```python
from build123d import *

# Parameters (mm, degrees)
F0_W     = 50.8
F0_H     = 50.8
F1_DEPTH = 50.8
F3_DEPTH = 25.4
F4_R     = 12.7
F5_DEPTH = 25.4
F6_R     = 12.7
F7_DEPTH = 25.4


with BuildPart() as f1:
    # F0 (on Front) → F1 (new body)
    with BuildSketch(Plane.XZ):
        with Locations((-25.4, 25.4)):
            Rectangle(F0_W, F0_H)
    extrude(amount=F1_DEPTH)

    # F2 (on face) → F3 (join)
    with BuildSketch(Plane.XZ.offset(50.8)):
        Polygon((-12.7, 38.1), (-38.1, 38.1), (-38.1, 10.884415), (-12.984917, 10.884415), align=None)
    extrude(amount=F3_DEPTH)

    # F4 (on face) → F5 (join)
    with BuildSketch(Plane.YZ):
        with Locations((-25.738167, 25.206015)):
            Circle(F4_R)
    extrude(amount=F5_DEPTH)

    # F6 (on face) → F7 (cut)
    with BuildSketch(Plane.XY.offset(50.8)):
        with Locations((-25.587924, -25.396967)):
            Circle(F6_R)
    extrude(amount=-F7_DEPTH, mode=Mode.SUBTRACT)


solid = f1.part
```
CAD build for the part. Positions are in the model's coordinates, mm. A direction names the side the tool comes from. Coordinates: 2 decimals unless noted, no trailing zeros. Order: outer loops, then holes, each group sorted by start corner. A loop starts at its lowest first (then second) coordinate and runs counter-clockwise, first axis right, second up. Notation, with made-up numbers: (16, 34) - (68, 34) arc R13 cw to (68, 54) - close; hole circle Ø9 at (36.5, 73.5). An arc over 180 degrees is marked (long way). Answer in a Markdown table with one row per item.
1. Slice it at D-D, the plane z = 15.5. List the corners of the cut face in (x, y).
Answer:
| item | result |
|---|---|
| outline | (-50.8, -50.8) - (-38.1, -50.8) - (-38.1, -76.2) - (-12.94, -76.2) - (-12.94, -50.8) - (0, -50.8) - (0, -33.93) - (25.4, -33.93) - (25.4, -17.55) - (0, -17.55) - (0, 0) - (-50.8, 0) - close |
2. Flat gauge pins, fed straight in: P1, Ø7.5, axis at x = -27, y = -66.5, coming from the +Z side; P2, Ø4, axis at x = -9, z = 12, coming from the -Y side; P3, Ø1.5, axis at x = 11.5, y = -25, coming from the -Z side. Where does each tip first touch, or does it go through?
Answer:
| item | result |
|---|---|
| P1 | z = 38.1 |
| P2 | y = -50.8 |
| P3 | z = 12.51 |
3. 3-axis set-ups, long thin cutter, end or side, ignore diameter. For faces 1 (the face through (-38.1, -63, 25)), 2 (the face through (-26, -63, 10.884)), 3 (the face through (-31.4, -13.8, 50.8)), 4 (the face through (-26, -25, 25.4)), 5 (the face through (0, -14, 31)): which of +Z, -Z, +X, -X, +Y, -Y reach the whole face in a straight line?
Answer:
| item | result |
|---|---|
| face 1 | +Z, -Z, -X, -Y |
| face 2 | -Z, +X, -X, -Y |
| face 3 | +Z, +X, -X, +Y, -Y |
| face 4 | +Z |
| face 5 | +X |
4. Drill centre lines: L1, parallel to Y at x = -8, z = 2.5; L2, parallel to X at y = -21, z = 39. Where is each one in solid material? Low to high. Write a range as from..to.
Answer:
| item | result |
|---|---|
| L1 | -50.8..0 |
| L2 | -50.8..-37.5, -13.67..0 |
5. Pull direction X, two halves, no side cores. Call faces 6 (the face through (-25, -63, 38.1)), 7 (the face through (-34.948, -16.814, 38.278)), 8 (the face through (25.4, -26, 25)): +X half, -X half, draft (parallel to the pull), parting line (faces both ways), or undercut.
Answer:
| item | result |
|---|---|
| face 6 | draft |
| face 7 | undercut |
| face 8 | +X half |
6. Slice it at A-A, the plane z = 35. List the corners of the cut face in (x, y), then the cut area to 3 significant figures.
Answer:
| item | result |
|---|---|
| outline | (-50.8, -50.8) - (-38.1, -50.8) - (-38.1, -76.2) - (-12.73, -76.2) - (-12.73, -50.8) - (0, -50.8) - (0, -33.82) - (25.4, -33.82) - (25.4, -17.65) - (0, -17.65) - (0, 0) - (-50.8, 0) - close; hole circle Ø25.4 at (-25.59, -25.4) |
| area | 3,130 mm² |
7. Slice it at B-B, the plane y = -71. List the corners of the cut face in (x, z).
Answer:
| item | result |
|---|---|
| outline | (-38.1, 10.88) - (-12.98, 10.88) - (-12.7, 38.1) - (-38.1, 38.1) - close |
8. Slice it at C-C, the plane x = -30.5. List the corners of the cut face in (y, z), then the cut area to 3 significant figures.
Answer:
| item | result |
|---|---|
| outline | (-76.2, 10.88) - (-50.8, 10.88) - (-50.8, 0) - (0, 0) - (0, 50.8) - (-13.69, 50.8) - (-13.69, 25.4) - (-37.11, 25.4) - (-37.11, 50.8) - (-50.8, 50.8) - (-50.8, 38.1) - (-76.2, 38.1) - close |
| area | 2,680 mm² |
